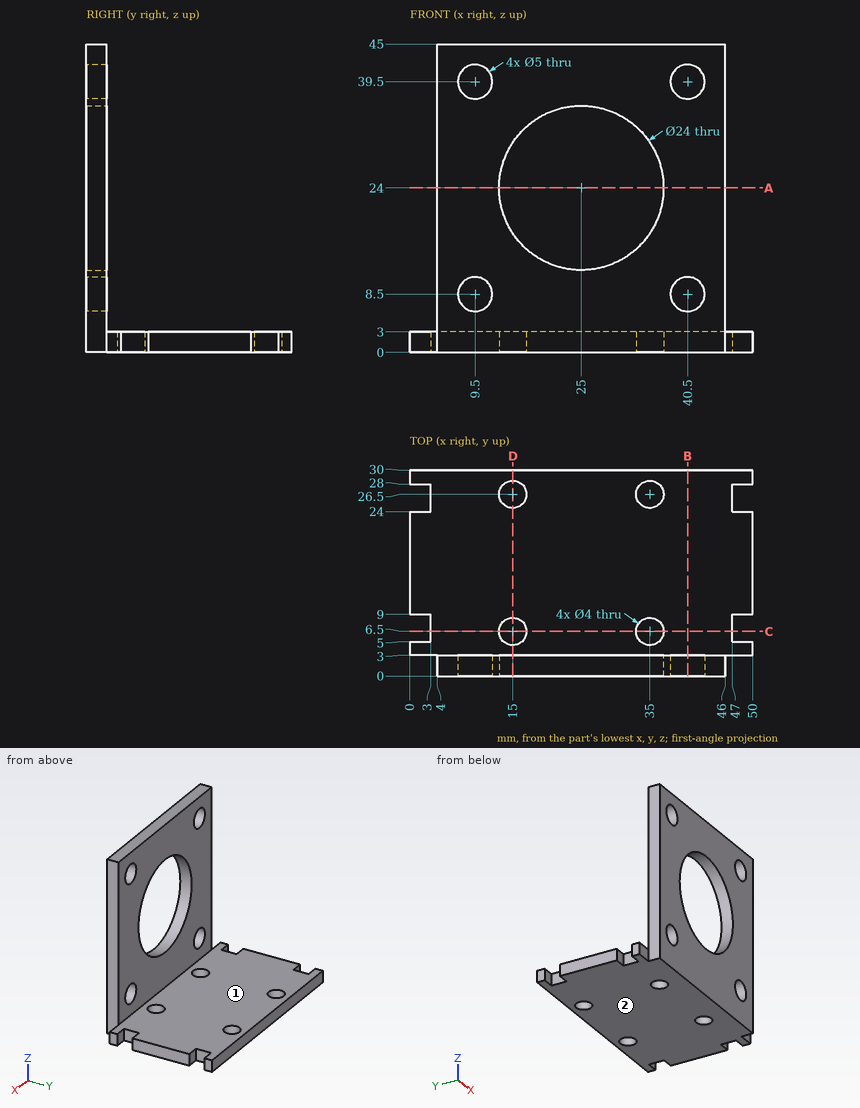
Source: three-view drawing plus pictorial views. Frame: mm from the lowest corner of the part. A direction names the side the tool comes from. Give positions to 0.01 mm unless a question says otherwise; leave off trailing zeros. Order: outer loops, then holes, each group sorted by start corner. A loop starts at its lowest first (then second) coordinate and runs counter-clockwise, first axis right, second up.
1. Section B-B on x = 40.5. Return the cut outline in (y, z).
Derived:
outline: (0, 0) - (30, 0) - (30, 3) - (3, 3) - (3, 6) - (0, 6) - close; (0, 11) - (3, 11) - (3, 37) - (0, 37) - close; (0, 42) - (3, 42) - (3, 45) - (0, 45) - close
2. Section D-D on x = 15. Return the cut outline in (y, z), and give its area (3 significant figures).
Derived:
outline: (0, 0) - (4.5, 0) - (4.5, 3) - (3, 3) - (3, 17.37) - (0, 17.37) - close; (0, 30.63) - (3, 30.63) - (3, 45) - (0, 45) - close; (8.5, 0) - (24.5, 0) - (24.5, 3) - (8.5, 3) - close; (28.5, 0) - (30, 0) - (30, 3) - (28.5, 3) - close
area: 152 mm2
3. Reachability of the marked faces 1 and 2 from +Z, -Z, +X, -X, +Y, -Y: full face, straight path, thin tool, end or side. Return the list, or none.
Derived:
face 1: +Z, +X, -X, +Y
face 2: -Z, +X, -X, +Y, -Y
4. Pin query (flat end, axial travel): pin 1 (5 mm diameter, centred on x = 31.5, z = 14, fed in from +Y); pin 2 (0.9 mm diameter, centred on y = 26.5, z = 1, fed in from +X); pin 3 (0.9 mm diameter, centred on x = 2, z = 1.5, fed in from -Y); pin 4 (3 mm diameter, centred on x = 35, y = 6.5, fed in from +Z). Return the tip coordinate at first contact, or that it passes through.
Derived:
pin 1: stops at y = 3
pin 2: stops at x = 47
pin 3: stops at y = 3
pin 4: passes through
5. Section A-A on z = 24. Return the cut outline in (x, y), and give its area (3 significant figures).
Derived:
outline: (4, 0) - (13, 0) - (13, 3) - (4, 3) - close; (37, 0) - (46, 0) - (46, 3) - (37, 3) - close
area: 54.0 mm2
6. Section C-C on y = 6.5. Return the cut outline in (x, z).
Derived:
outline: (3, 0) - (13, 0) - (13, 3) - (3, 3) - close; (17, 0) - (33, 0) - (33, 3) - (17, 3) - close; (37, 0) - (47, 0) - (47, 3) - (37, 3) - close
7. Material intervals for L1, parallel to Z at x = 9.5, y = 0.9; L2, parallel to Y at x = 35, z = 1.3; L3, parallel to Z at x = 25, y = 0.85, sorted ascending.
Derived:
L1: z = 0 to 6, 11 to 37, 42 to 45
L2: y = 0 to 4.5, 8.5 to 24.5, 28.5 to 30
L3: z = 0 to 12, 36 to 45
